```python
from build123d import *

# Parameters (mm, degrees)
SKETCH1_R           = 17.5
BOSS_EXTRUDE1_DEPTH = 10.25
SKETCH2_R           = 2.5
BOSS_EXTRUDE2_DEPTH = 0.5
SKETCH3_R           = 2.5
BOSS_EXTRUDE3_DEPTH = 0.5
CIRPATTERN1_COUNT   = 4


with BuildPart() as part:
    # Sketch1 → Boss-Extrude1 (new, symmetric)
    with BuildSketch(Plane.XY):
        with BuildLine():
            Line((-5, 20.645822822), (-5, 36.945906404))
            ThreePointArc((-5, 36.945906404), (-4.177898814, 39.00909732), (-2.162162162, 39.941520437))
            ThreePointArc((-2.162162162, 39.941520437), (0, 40), (2.162162162, 39.941520437))
            ThreePointArc((2.162162162, 39.941520437), (4.177898814, 39.00909732), (5, 36.945906404))
            Line((5, 36.945906404), (5, 20.645822822))
            ThreePointArc((5, 20.645822822), (5.200290751, 20.04543535), (5.720930233, 19.685551993))
            ThreePointArc((5.720930233, 19.685551993), (7.845010363, 18.939530416), (9.874478744, 17.965095868))
            ThreePointArc((9.874478744, 17.965095868), (10.497102414, 17.851424122), (11.063267415, 18.134335227))
            Line((11.063267415, 18.134335227), (22.589167049, 29.660234861))
            ThreePointArc((22.589167049, 29.660234861), (24.629376661, 30.537817825), (26.714040425, 29.771799478))
            ThreePointArc((26.714040425, 29.771799478), (28.284271247, 28.284271247), (29.771799478, 26.714040425))
            ThreePointArc((29.771799478, 26.714040425), (30.537817825, 24.629376661), (29.660234861, 22.589167049))
            Line((29.660234861, 22.589167049), (18.134335227, 11.063267415))
            ThreePointArc((18.134335227, 11.063267415), (17.851424122, 10.497102414), (17.965095868, 9.874478744))
            ThreePointArc((17.965095868, 9.874478744), (18.939530416, 7.845010363), (19.685551993, 5.720930233))
            ThreePointArc((19.685551993, 5.720930233), (20.04543535, 5.200290751), (20.645822822, 5))
            Line((20.645822822, 5), (36.945906404, 5))
            ThreePointArc((36.945906404, 5), (39.00909732, 4.177898814), (39.941520437, 2.162162162))
            ThreePointArc((39.941520437, 2.162162162), (40, 0), (39.941520437, -2.162162162))
            ThreePointArc((39.941520437, -2.162162162), (39.00909732, -4.177898814), (36.945906404, -5))
            Line((36.945906404, -5), (20.645822822, -5))
            ThreePointArc((20.645822822, -5), (20.04543535, -5.200290751), (19.685551993, -5.720930233))
            ThreePointArc((19.685551993, -5.720930233), (18.939530416, -7.845010363), (17.965095868, -9.874478744))
            ThreePointArc((17.965095868, -9.874478744), (17.851424122, -10.497102414), (18.134335227, -11.063267415))
            Line((18.134335227, -11.063267415), (29.660234861, -22.589167049))
            ThreePointArc((29.660234861, -22.589167049), (30.537817825, -24.629376661), (29.771799478, -26.714040425))
            ThreePointArc((29.771799478, -26.714040425), (28.284271247, -28.284271247), (26.714040425, -29.771799478))
            ThreePointArc((26.714040425, -29.771799478), (24.629376661, -30.537817825), (22.589167049, -29.660234861))
            Line((22.589167049, -29.660234861), (11.063267415, -18.134335227))
            ThreePointArc((11.063267415, -18.134335227), (10.497102414, -17.851424122), (9.874478744, -17.965095868))
            ThreePointArc((9.874478744, -17.965095868), (7.845010363, -18.939530416), (5.720930233, -19.685551993))
            ThreePointArc((5.720930233, -19.685551993), (5.200290751, -20.04543535), (5, -20.645822822))
            Line((5, -20.645822822), (5, -36.945906404))
            ThreePointArc((5, -36.945906404), (4.177898814, -39.00909732), (2.162162162, -39.941520437))
            ThreePointArc((2.162162162, -39.941520437), (0, -40), (-2.162162162, -39.941520437))
            ThreePointArc((-2.162162162, -39.941520437), (-4.177898814, -39.00909732), (-5, -36.945906404))
            Line((-5, -36.945906404), (-5, -20.645822822))
            ThreePointArc((-5, -20.645822822), (-5.200290751, -20.04543535), (-5.720930233, -19.685551993))
            ThreePointArc((-5.720930233, -19.685551993), (-7.845010363, -18.939530416), (-9.874478744, -17.965095868))
            ThreePointArc((-9.874478744, -17.965095868), (-10.497102414, -17.851424122), (-11.063267415, -18.134335227))
            Line((-11.063267415, -18.134335227), (-22.589167049, -29.660234861))
            ThreePointArc((-22.589167049, -29.660234861), (-24.629376661, -30.537817825), (-26.714040425, -29.771799478))
            ThreePointArc((-26.714040425, -29.771799478), (-28.284271247, -28.284271247), (-29.771799478, -26.714040425))
            ThreePointArc((-29.771799478, -26.714040425), (-30.537817825, -24.629376661), (-29.660234861, -22.589167049))
            Line((-29.660234861, -22.589167049), (-18.134335227, -11.063267415))
            ThreePointArc((-18.134335227, -11.063267415), (-17.851424122, -10.497102414), (-17.965095868, -9.874478744))
            ThreePointArc((-17.965095868, -9.874478744), (-18.939530416, -7.845010363), (-19.685551993, -5.720930233))
            ThreePointArc((-19.685551993, -5.720930233), (-20.04543535, -5.200290751), (-20.645822822, -5))
            Line((-20.645822822, -5), (-36.945906404, -5))
            ThreePointArc((-36.945906404, -5), (-39.00909732, -4.177898814), (-39.941520437, -2.162162162))
            ThreePointArc((-39.941520437, -2.162162162), (-40, 0), (-39.941520437, 2.162162162))
            ThreePointArc((-39.941520437, 2.162162162), (-39.00909732, 4.177898814), (-36.945906404, 5))
            Line((-36.945906404, 5), (-20.645822822, 5))
            ThreePointArc((-20.645822822, 5), (-20.04543535, 5.200290751), (-19.685551993, 5.720930233))
            ThreePointArc((-19.685551993, 5.720930233), (-18.939530416, 7.845010363), (-17.965095868, 9.874478744))
            ThreePointArc((-17.965095868, 9.874478744), (-17.851424122, 10.497102414), (-18.134335227, 11.063267415))
            Line((-18.134335227, 11.063267415), (-29.660234861, 22.589167049))
            ThreePointArc((-29.660234861, 22.589167049), (-30.537817825, 24.629376661), (-29.771799478, 26.714040425))
            ThreePointArc((-29.771799478, 26.714040425), (-28.284271247, 28.284271247), (-26.714040425, 29.771799478))
            ThreePointArc((-26.714040425, 29.771799478), (-24.629376661, 30.537817825), (-22.589167049, 29.660234861))
            Line((-22.589167049, 29.660234861), (-11.063267415, 18.134335227))
            ThreePointArc((-11.063267415, 18.134335227), (-10.497102414, 17.851424122), (-9.874478744, 17.965095868))
            ThreePointArc((-9.874478744, 17.965095868), (-7.845010363, 18.939530416), (-5.720930233, 19.685551993))
            ThreePointArc((-5.720930233, 19.685551993), (-5.200290751, 20.04543535), (-5, 20.645822822))
        make_face()
        Circle(SKETCH1_R, mode=Mode.SUBTRACT)
    extrude(amount=BOSS_EXTRUDE1_DEPTH, both=True)

    # Sketch2 → Boss-Extrude2 (add, symmetric)
    with BuildSketch(Plane.XY.offset(10.25)):
        with Locations(Location((0, 30, 0), (0, 0, 180))):
            Circle(SKETCH2_R)
    boss_extrude2 = extrude(amount=BOSS_EXTRUDE2_DEPTH, both=True)

    # Sketch3 → Boss-Extrude3 (add, symmetric)
    with BuildSketch(Plane(origin=(0, 0, -10.25), x_dir=(-1, 0, 0), z_dir=(0, 0, -1))):
        with Locations((-21.213203436, 21.213203436)):
            Circle(SKETCH3_R)
    boss_extrude3 = extrude(amount=BOSS_EXTRUDE3_DEPTH, both=True)

    # CirPattern1: Boss-Extrude2, Boss-Extrude3 ×4 about axis
    cirpattern1_axis = Axis((0, 0, 0), (0, 0, 1))
    add([boss_extrude2.rotate(cirpattern1_axis, i * 360 / CIRPATTERN1_COUNT) for i in range(1, CIRPATTERN1_COUNT)])
    add([boss_extrude3.rotate(cirpattern1_axis, i * 360 / CIRPATTERN1_COUNT) for i in range(1, CIRPATTERN1_COUNT)])


solid = part.part
```
The model under review builds one solid part; all positions refer to its coordinate system, in mm. A direction names the side the tool comes from. Coordinates: 2 decimals unless noted, no trailing zeros. Loops run counter-clockwise (first coordinate to the right, second up) from the corner with the lowest first, then second, coordinate; pieces in that order, holes last. Notation, with made-up numbers: (42.25, 70.5) -> (65.25, 70.5) arc R29 cw to (65.25, 100.5) -> close; hole circle Ø10 at (87.25, 40). An arc over 180 degrees is marked (long way). Answer as CSV lines item,"result".
Item 1: Machinability: for faces 4 (the cylindrical face through (-27.52, 0.33, 10.5)), 5 (the cylindrical face through (18.95, -7.82, 0.14)), 6 (the cylindrical face through (-22.9, 23.06, -10.5)), which of the approach directions +Z, -Z, +X, -X, +Y, -Y give a long, thin tool a straight path to every point of the face, cutting with its end or side? Answer none if there is none.
Results below:
face 4,"+Z"
face 5,"+Z, -Z, +X"
face 6,"-Z"
Item 2: For L1, parallel to Y at x = -21, z = 1.25; L2, parallel to Y at x = 27.5, z = -1.25; L3, parallel to X at y = 3, z = 8, list the stretches that pass through material, from the lowest coordinate up.
Results below:
L1,"y = -28.07 to -13.93, -5 to 5, 13.93 to 28.07"
L2,"y = -29.05 to -20.43, -5 to 5, 20.43 to 29.05"
L3,"x = -39.77 to -17.24, 17.24 to 39.77"
Item 3: Take a section at A-A, the plane x = 0. State the section outline as (y, z) points, and give its area (4 significant figures).
Results below:
outline,"(-40, -10.25) -> (-17.5, -10.25) -> (-17.5, 10.25) -> (-27.5, 10.25) -> (-27.5, 10.75) -> (-32.5, 10.75) -> (-32.5, 10.25) -> (-40, 10.25) -> close; (17.5, -10.25) -> (40, -10.25) -> (40, 10.25) -> (32.5, 10.25) -> (32.5, 10.75) -> (27.5, 10.75) -> (27.5, 10.25) -> (17.5, 10.25) -> close"
area,"927.5 mm2"
Item 4: Take a section at C-C, the plane x = -12. State the section outline as (y, z) points, and give its area (3 significant figures).
Results below:
outline,"(-19.07, -10.25) -> (-12.74, -10.25) -> (-12.74, 10.25) -> (-19.07, 10.25) -> close; (12.74, -10.25) -> (19.07, -10.25) -> (19.07, 10.25) -> (12.74, 10.25) -> close"
area,"260 mm2"
Item 5: Insertion check: pin 1 (5 mm diameter, centred on x = -26, z = 3, fed in from -Y); pin 2 (6 mm diameter, centred on x = 7, y = 19.5, fed in from +Z); pin 3 (8 mm diameter, centred on y = -31.5, z = 3, fed in from -X); pin 4 (12 mm diameter, centred on x = 0.5, z = -2, fed in from +Y). Each pin has a flat end and moves straight along its axis. Give the tip position at first contact, or say it passes through.
Results below:
pin 1,"stops at y = -30.54"
pin 2,"stops at z = 10.25"
pin 3,"stops at x = -29.05"
pin 4,"stops at y = 40"
Item 6: Draft analysis for pull direction Y (two halves, no side actions). For faces 1 (the flat face through (-23.82, 16.75, 0.14)), 2 (the cylindrical face through (27.52, -0.33, 10.5)), 3 (the cylindrical face through (-24.598, -30.537, 0.143)), state which applies: +Y half, -Y half, draft (parallel to the pull), parting line (faces both ways), or undercut.
Results below:
face 1,"undercut"
face 2,"parting line"
face 3,"-Y half"
Item 7: Take a section at B-B, the plane y = -8.5. State the section outline as (x, z) points.
Results below:
outline,"(-18.65, -10.25) -> (-15.3, -10.25) -> (-15.3, 10.25) -> (-18.65, 10.25) -> close; (15.3, -10.25) -> (18.65, -10.25) -> (18.65, 10.25) -> (15.3, 10.25) -> close"
